Autodesk Inventor part; units mm, degrees
ref_plane "YZ Plane" through (0, 0, 0) normal (1, 0, 0) x (0, 1, 0)
ref_plane "XZ Plane" through (0, 0, 0) normal (0, 1, 0) x (-1, 0, 0)
ref_plane "XY Plane" through (0, 0, 0) normal (0, 0, 1) x (1, 0, 0)
sketch "스케치1" plane through (0, 0, 0) normal (0, 1, 0) x (-1, 0, 0)
  line L0 (22, -14) -> (-22, -14)
  line L1 (-22, -14) -> (-22, 14)
  line L2 (-22, 14) -> (22, 14)
  line L3 (22, 14) -> (22, -14)
  point P0 (0, 0)
  dimension "d0" = 44
  dimension "d1" = 22
  dimension "d2" = 28
  dimension "d3" = 14
extrude "돌출1" add sketch "스케치1" along normal blind 5
sketch "스케치2" plane through (-22, 0, 14) normal (0, 0, 1) x (1, 0, 0)
  circle A0 centre (33, 3) radius 1.5
  circle A1 centre (11, 3) radius 1.5
  line L0 (44, 0) -> (0, 0)
  line L1 (22, 0) -> (22, 5)
  line L2 (44, 5) -> (0, 5)
  dimension "d6" = 3
  dimension "d7" = 3
  dimension "d8" = 3
  dimension "d9" = 3
  dimension "d10" = 22
  dimension "d11" = 11
extrude "돌출2" cut sketch "스케치2" against normal blind 60
sketch "스케치3" plane through (0, 0, 0) normal (0, -1, 0) x (1, 0, 0)
  line L0 (-17, 14.5) -> (17, 14.5)
  line L1 (17, 14.5) -> (17, -14.5)
  line L2 (17, -14.5) -> (-17, -14.5)
  line L3 (-17, -14.5) -> (-17, 14.5)
  line L4 (22, -14) -> (-22, -14)
  line L5 (22, 25.1) -> (-22, 25.1)
  line L6 (-22, 25.1) -> (-22, -25.1)
  line L7 (-22, -25.1) -> (22, -25.1)
  line L8 (22, -25.1) -> (22, 25.1)
  point P0 (0, 0)
  dimension "d17" = 34
  dimension "d18" = 17
  dimension "d20" = 29
  dimension "d21" = 14.5
  dimension "d22" = 10.6
  dimension "d23" = 10.6
  dimension "d24" = 5
  dimension "d25" = 5
extrude "돌출3" add sketch "스케치3" along normal blind 2
sketch "스케치4" plane through (0, -2, 0) normal (0, -1, 0) x (1, 0, 0)
  line L0 (-22, 25.1) -> (-22, -25.1)
  line L1 (-22, -25.1) -> (22, -25.1)
  line L2 (-22, 25.1) -> (22, 25.1)
  line L3 (22, 25.1) -> (22, -25.1)
  line L4 (22, -25.1) -> (-22, -25.1)
  line L5 (-22, -25.1) -> (-22, 25.1)
  line L6 (-17, 20.1) -> (17, 20.1)
  line L7 (17, 20.1) -> (17, -20.1)
  line L8 (17, -20.1) -> (-17, -20.1)
  line L9 (-17, -20.1) -> (-17, 20.1)
  point P0 (0, 0)
  dimension "d28" = 5
  dimension "d29" = 5
  dimension "d30" = 5
  dimension "d31" = 5
extrude "돌출4" add sketch "스케치4" along normal blind 5.58
sketch "스케치5" plane through (22, 5, 14) normal (1, 0, 0) x (0, 0, -1)
  circle A0 centre (25, -9.8) radius 1.35
  circle A1 centre (3, -9.8) radius 1.35
  line L0 (39.1, -5) -> (28, -5)
  line L1 (0, -5) -> (-11.1, -5)
  point P0 (14, -5)
  dimension "d34" = 2.7
  dimension "d35" = 2.7
  dimension "d36" = 4.8
  dimension "d37" = 4.8
  dimension "d38" = 22
  dimension "d39" = 11
extrude "돌출5" cut sketch "스케치5" against normal blind 90
sketch "스케치6" plane through (0, -7.58, 0) normal (0, -1, 0) x (1, 0, 0)
  line L0 (22, -25.1) -> (-22, -25.1)
  line L1 (-22, -25.1) -> (-22, -20.1)
  line L2 (-22, -20.1) -> (22, -20.1)
  line L3 (22, -20.1) -> (22, -25.1)
  line L4 (22, 25.1) -> (-22, 25.1)
  line L5 (-22, 25.1) -> (-22, 20.1)
  line L6 (-22, 20.1) -> (22, 20.1)
  line L7 (22, 20.1) -> (22, 25.1)
  point P0 (0, 0)
  dimension "d42" = 5
  dimension "d43" = 5
extrude "돌출6" add sketch "스케치6" along normal blind 6
sketch "스케치7" plane through (0, -7.58, 0) normal (0, -1, 0) x (1, 0, 0)
  line L0 (22, -20.1) -> (-22, -20.1)
  line L1 (17, 20.1) -> (17, -20.1)
  line L2 (22, -20.1) -> (17, -20.1)
  line L3 (17, -20.1) -> (17, -14.6)
  line L4 (17, -14.6) -> (22, -14.6)
  line L5 (22, -14.6) -> (22, -20.1)
  line L6 (22, 14) -> (22, 25.1)
  line L7 (22, 20.1) -> (17, 20.1)
  line L8 (17, 20.1) -> (17, 14.6)
  line L9 (17, 14.6) -> (22, 14.6)
  line L10 (22, 14.6) -> (22, 20.1)
  line L11 (-22, -14) -> (-22, 14)
  line L12 (-17, -20.1) -> (-22, -20.1)
  line L13 (-22, -20.1) -> (-22, -14.6)
  line L14 (-22, -14.6) -> (-17, -14.6)
  line L15 (-17, -14.6) -> (-17, -20.1)
  line L16 (-17, 20.1) -> (-22, 20.1)
  line L17 (-22, 20.1) -> (-22, 14.6)
  line L18 (-22, 14.6) -> (-17, 14.6)
  line L19 (-17, 14.6) -> (-17, 20.1)
  line L20 (22, 20.1) -> (17, 20.1)
  point P0 (0, 0)
  dimension "d46" = 5.5
  dimension "d47" = 5.5
  dimension "d48" = 5.5
  dimension "d49" = 5.5
  dimension "d50" = 0
extrude "돌출7" add sketch "스케치7" along normal blind 55.52
sketch "스케치8" plane through (0, -13.58, 0) normal (0, -1, 0) x (1, 0, 0)
  line L0 (-22, -20.1) -> (-22, -25.1)
  line L1 (-17, -20.1) -> (-22, -20.1)
  line L2 (-22, -25.1) -> (-17, -25.1)
  line L3 (-17, -25.1) -> (-17, -20.1)
  line L4 (-17, -20.1) -> (-22, -20.1)
  line L5 (-22, -20.1) -> (-22, -25.1)
  line L6 (-17, -20.1) -> (17, -20.1)
  line L7 (22, -25.1) -> (22, -20.1)
  line L8 (17, -20.1) -> (22, -20.1)
  line L9 (22, -20.1) -> (22, -25.1)
  line L10 (22, -25.1) -> (17, -25.1)
  line L11 (17, -25.1) -> (17, -20.1)
  line L12 (17, -20.1) -> (17, 20.1)
  line L13 (22, 20.1) -> (22, 25.1)
  line L14 (17, 20.1) -> (22, 20.1)
  line L15 (22, 20.1) -> (22, 25.1)
  line L16 (22, 25.1) -> (17, 25.1)
  line L17 (17, 25.1) -> (17, 20.1)
  line L18 (-22, 25.1) -> (-22, 20.1)
  line L19 (22, 25.1) -> (-22, 25.1)
  line L20 (-22, 20.1) -> (-17, 20.1)
  line L21 (-17, 20.1) -> (-17, 25.1)
  line L22 (-17, 25.1) -> (-22, 25.1)
  line L23 (-22, 25.1) -> (-22, 20.1)
  point P0 (0, 0)
extrude "돌출8" add sketch "스케치8" along normal blind 49.52
sketch "스케치9" plane through (-22, 5, -14) normal (-1, 0, 0) x (0, 0, 1)
  circle A0 centre (31.3, -59.1) radius 1.35
  circle A1 centre (-3.3, -59.1) radius 1.35
  line L0 (-0.6, -68.1) -> (-11.1, -68.1)
  line L1 (39.1, -68.1) -> (28.6, -68.1)
  line L2 (39.1, -5) -> (39.1, -68.1)
  line L3 (-11.1, -5) -> (-11.1, -68.1)
  circle A2 centre (31.3, -37.1) radius 1.35
  circle A3 centre (-3.3, -37.1) radius 1.35
  point P0 (14, -5)
  dimension "d55" = 9
  dimension "d56" = 9
  dimension "d57" = 2.7
  dimension "d58" = 2.7
  dimension "d59" = 7.8
  dimension "d60" = 7.8
  dimension "d61" = 2.7
  dimension "d62" = 2.7
  dimension "d63" = 22
  dimension "d64" = 22
extrude "돌출9" cut sketch "스케치9" against normal blind 49.52
sketch "스케치11" plane through (-22, 5, -14) normal (-1, 0, 0) x (0, 0, 1)
  line L0 (28, 0) -> (0, 0)
  line L1 (0, -5) -> (-11.1, -5)
  line L2 (28, 0) -> (0, 0)
  line L3 (0, 0) -> (0, -5)
  line L4 (0, -5) -> (28, -5)
  line L5 (28, -5) -> (28, 0)
  point P0 (14, -5)
extrude "돌출11" cut sketch "스케치11" against normal blind 80
sketch "스케치14" plane through (-22, 0, -25.1) normal (-1, 0, 0) x (0, 0, 1)
  line L0 (0, -63.1) -> (10.5, -63.1)
  line L1 (0, -63.1) -> (10.5, -63.1)
  line L2 (10.5, -7.58) -> (10.5, -63.1)
  line L3 (10.5, -63.1) -> (10.5, -7.58)
  line L4 (10.5, -7.58) -> (39.7, -7.58)
  line L5 (39.7, -7.58) -> (39.7, -63.1)
  line L6 (39.7, -7.58) -> (39.7, -63.1)
  line L7 (39.7, -63.1) -> (50.2, -63.1)
  line L8 (39.7, -63.1) -> (50.2, -63.1)
  line L9 (50.2, 0) -> (50.2, -63.1)
  line L10 (50.2, -63.1) -> (50.2, 0)
  line L11 (50.2, 0) -> (0, 0)
  line L12 (50.2, 0) -> (0, 0)
  line L13 (0, -13.58) -> (0, -63.1)
  line L14 (0, 0) -> (0, -63.1)
  point P0 (25.1, 0)
extrude "돌출14" add sketch "스케치14" along normal blind 10
sketch "스케치15" plane through (-17, -63.1, 14.6) normal (0, 0, -1) x (-1, 0, 0)
  line L0 (15, 55.52) -> (15, 0)
  line L1 (0, 55.52) -> (15, 55.52)
  line L2 (15, 0) -> (10, 0)
  line L3 (10, 0) -> (10, 55.52)
  line L4 (10, 55.52) -> (15, 55.52)
  line L5 (15, 55.52) -> (15, 0)
  point P0 (-17, 63.1)
  dimension "d86" = 5
extrude "돌출15" add sketch "스케치15" along normal blind 0.4
sketch "스케치16" plane through (-17, -63.1, -14.6) normal (0, 0, 1) x (1, 0, 0)
  line L0 (-15, 0) -> (-15, 55.52)
  line L1 (-15, 55.52) -> (0, 55.52)
  line L2 (-15, 0) -> (-10, 0)
  line L3 (-10, 0) -> (-10, 55.52)
  line L4 (-10, 55.52) -> (-15, 55.52)
  line L5 (-15, 55.52) -> (-15, 0)
  point P0 (17, 63.1)
  dimension "d89" = 5
extrude "돌출16" add sketch "스케치16" along normal blind 0.4
sketch "스케치17" plane through (17, -13.58, -25.1) normal (0, 0, -1) x (-1, 0, 0)
  line L0 (13.776, -36.52) -> (66.3511, -36.52)
  line L1 (34, -49.52) -> (49, -49.52)
  circle A0 centre (46, -47.52) radius 1.5
  circle A1 centre (46, -25.52) radius 1.5
  line L2 (49, 13.58) -> (49, -49.52)
  point P0 (17, 13.58)
  dimension "d92" = 13
  dimension "d93" = 3
  dimension "d94" = 3
  dimension "d95" = 3
  dimension "d96" = 3
  dimension "d97" = 22
  dimension "d98" = 11
extrude "돌출17" cut sketch "스케치17" against normal blind 100
sketch "스케치18" plane through (0, -63.1, 0) normal (0, -1, 0) x (1, 0, 0)
  line L0 (-17, 25.1) -> (-17, 20.1)
  line L1 (-17, 14.6) -> (-27, 14.6)
  line L2 (-17, 25.1) -> (-27, 25.1)
  line L3 (-27, 25.1) -> (-27, 14.6)
  line L4 (-27, 14.6) -> (-17, 14.6)
  line L5 (-17, 14.6) -> (-17, 25.1)
  line L6 (-27, 14.2) -> (-32, 14.2)
  line L7 (-27, 25.1) -> (-32, 25.1)
  line L8 (-32, 25.1) -> (-32, 14.2)
  line L9 (-32, 14.2) -> (-27, 14.2)
  line L10 (-27, 14.2) -> (-27, 25.1)
  line L11 (-27, -14.6) -> (-17, -14.6)
  line L12 (22, -25.1) -> (-32, -25.1)
  line L13 (-17, -14.6) -> (-27, -14.6)
  line L14 (-27, -14.6) -> (-27, -25.1)
  line L15 (-27, -25.1) -> (-17, -25.1)
  line L16 (-17, -25.1) -> (-17, -14.6)
  line L17 (-32, -14.2) -> (-27, -14.2)
  line L18 (-32, 25.1) -> (-32, -25.1)
  line L19 (-27, -14.2) -> (-32, -14.2)
  line L20 (-32, -14.2) -> (-32, -25.1)
  line L21 (-32, -25.1) -> (-27, -25.1)
  line L22 (-27, -25.1) -> (-27, -14.2)
  point P0 (0, 0)
extrude "돌출18" add sketch "스케치18" along normal blind 5
properties part number "elbow_fore"
Read the model definition and answer for the solid it produces. Units are mm, in the model's axes. A direction names the side the tool comes from. Coordinates: 2 decimals unless noted, no trailing zeros. Order: outer loops, then holes, each group sorted by start corner. A loop starts at its lowest first (then second) coordinate and runs counter-clockwise, first axis right, second up. Notation, with made-up numbers: M 83.5,-25 L 120.5,-25 A23 cw 120.5,-13 Z; hole C 83,79.5 d8. An arc over 180 degrees is marked long. Put each result on its own line as item: value. Start each with the question number.
Item 1: For faces 4 (the face through (19, -35, -14.6)), 5 (the face through (0, -13.58, -23)), 6 (the face through (-19.535, -31.694, -16.012)), 7 (the face through (-25, -68.1, -20)), 8 (the face through (19, -63.1, 20)), determine the directions among +Z, -Z, +X, -X, +Y, -Y from which every point of the face is accessible in a straight line to the end or side of a thin tool.
Item 2: Section C-C, the plane y = -61.1 is taken. Determine the outline of the cut face in (x, z).
Item 3: Consider probe 1 along Z at (x, y) = (20, -32); probe 2 along Y at (x, z) = (20.6, -17.3); probe 3 along Z at (x, y) = (-27.5, -51.5). Determine where each line is inside the solid, lowest interval first. Write a range as [from, to].
Item 4: Section A-A, the plane y = -23 is taken. Determine the outline of the cut face in (x, z).
Item 5: Section D-D, the plane x = 5 is taken. Determine the outline of the cut face in (y, z).
Item 6: Section B-B, the plane z = -17.3 is taken. Determine the outline of the cut face in (x, y), plus the area to 3 significant figures.
Item 7: The mould has two halves that part along X. Classify faces 1 (the face through (-22, -54, -17)), 2 (the face through (-19.535, -52.761, 17.124)), 3 (the face through (0, -8, 20.1)): +X half, -X half, draft (parallel to the pull), parting line (faces both ways), or undercut.
Item 8: Given pin 1 Ø1.6 at (y, z) = (-32.1, 17.3) entering from +X; pin 2 Ø12 at (x, y) = (-7.5, -29) entering from +Z; pin 3 Ø5.5 at (x, z) = (20, 2.5) entering from -Y; pin 4 Ø4 at (x, z) = (15.5, -17.5) entering from -Y, each flat-ended and moving along its own axis, determine where each tip first touches the part or whether it passes through.
Computed:
1. face 4: +X, -Y
1. face 5: +Z, -Z, -Y
1. face 6: +X
1. face 7: +Z, -Z, +X, -X, -Y
1. face 8: +Z, -Z, +X, -Y
2. outline: M -32,-25.1 L -30.5,-25.1 L -30.5,-14.2 L -32,-14.2 Z; M -32,14.2 L -30.5,14.2 L -30.5,25.1 L -32,25.1 Z; M -27.5,-25.1 L -17,-25.1 L -17,-14.6 L -27,-14.6 L -27,-14.2 L -27.5,-14.2 Z; M -27.5,14.2 L -27,14.2 L -27,14.6 L -17,14.6 L -17,25.1 L -27.5,25.1 Z; M 17,-25.1 L 22,-25.1 L 22,-14.6 L 17,-14.6 Z; M 17,14.6 L 22,14.6 L 22,25.1 L 17,25.1 Z
3. probe 1: z = [-25.1, -18.65], [-15.95, -14.6], [14.6, 15.95], [18.65, 25.1]
3. probe 2: y = [-63.1, -55.45], [-52.75, -33.45], [-30.75, 0]
3. probe 3: z = [-25.1, -14.2], [14.2, 25.1]
4. outline: M -32,-25.1 L -17,-25.1 L -17,-14.6 L -27,-14.6 L -27,-14.2 L -32,-14.2 Z; M -32,14.2 L -27,14.2 L -27,14.6 L -17,14.6 L -17,25.1 L -32,25.1 Z; M 17,-25.1 L 22,-25.1 L 22,-14.6 L 17,-14.6 Z; M 17,14.6 L 22,14.6 L 22,25.1 L 17,25.1 Z
5. outline: M -13.58,-25.1 L 0,-25.1 L 0,25.1 L -13.58,25.1 L -13.58,20.1 L -2,20.1 L -2,-20.1 L -13.58,-20.1 Z
6. outline: M -32,-68.1 L -17,-68.1 L -17,-55.45 L -22,-55.45 L -22,-52.75 L -17,-52.75 L -17,-33.45 L -22,-33.45 L -22,-30.75 L -17,-30.75 L -17,-2 L 17,-2 L 17,-30.75 L 22,-30.75 L 22,0 L -32,0 Z; M 17,-63.1 L 22,-63.1 L 22,-55.45 L 17,-55.45 Z; M 17,-52.75 L 22,-52.75 L 22,-33.45 L 17,-33.45 Z; hole C -29,-61.1 d3; hole C -29,-39.1 d3
6. area: 1,340 mm2
7. face 1: +X half
7. face 2: draft
7. face 3: undercut
8. pin 1: stops at x = -22
8. pin 2: passes through
8. pin 3: stops at y = -7.58
8. pin 4: stops at y = -63.1
